Input: dimensioned drawing with shaded views. Units: mm. Origin: part minimum x, y, z. A direction names the side the tool comes from. Round coordinates to 2 decimals unless told otherwise and drop trailing zeros. Loops run counter-clockwise (first coordinate to the right, second up) from the corner with the lowest first, then second, coordinate; pieces in that order, holes last. Notation, with made-up numbers: M -10.5,-12.5 L 20.5,-12.5 A17 cw 20.5,18.5 Z; hole C -34,25 d1. An arc over 180 degrees is marked long. Use one line per item in the form item = value. Start each with the question number.
Q1. Section query A-A, the plane z = 5. Output: boundary loops of the cut face in (x, y).
Q2. Ray query, line 1 along X through (y, z) = (9.25, 6); line 2 along Z through (x, y) = (97.5, 4.75). Return the intervals inside material, ascending.
Q3. Section query C-C, the plane x = 72.5. Output: boundary loops of the cut face in (y, z), and give its area (3 significant figures).
Q4. First-contact query: P1, Ø2, axis at x = 60.5, y = 7, coming from the -Z side; P2, Ø5, axis at x = 60, z = 5, coming from the +Y side; P3, Ø1, axis at x = 14.5, z = 5.5, coming from the -Y side. Flat tips, straight axial feed; report the tip coordinate or a pass-through.
Q5. Access query for the marked faces 1 and 2. Directions: +Z, -Z, +X, -X, +Y, -Y. A direction counts if a zero-diameter tool reaches every point of the face in a straight line with its end or side. Return the directions, or none.
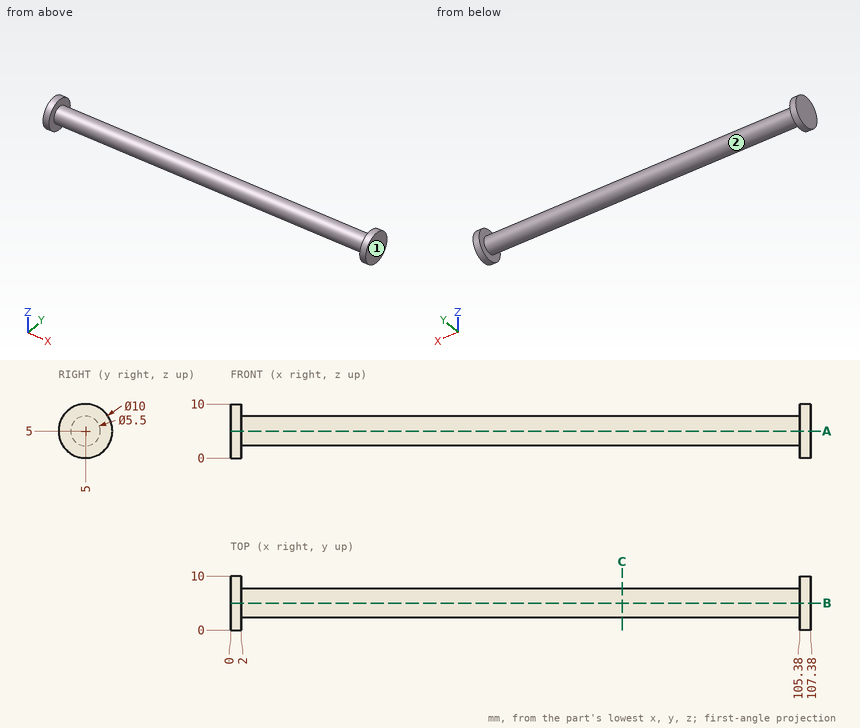
Results found:
q1.outline = M 0,0 L 2,0 L 2,2.25 L 105.38,2.25 L 105.38,0 L 107.38,0 L 107.38,10 L 105.38,10 L 105.38,7.75 L 2,7.75 L 2,10 L 0,10 Z
q2.line_1 = 0 to 2, 105.38 to 107.38
q2.line_2 = 2.26 to 7.74
q3.outline = C 5,5 d5.5
q3.area = 23.8 mm²
q4.P1 = 2.44
q4.P2 = 7.75
q4.P3 = 2.25
q5.face_1 = +Z, -Z, +X, +Y, -Y
q5.face_2 = none
